Autodesk Inventor part; units mm, degrees
ref_plane "YZ Plane" through (0, 0, 0) normal (1, 0, 0) x (0, 1, 0)
ref_plane "XZ Plane" through (0, 0, 0) normal (0, 1, 0) x (-1, 0, 0)
ref_plane "XY Plane" through (0, 0, 0) normal (0, 0, 1) x (1, 0, 0)
sketch "Sketch1" plane through (0, 0, 0) normal (0, 0, 1) x (1, 0, 0)
  line L0 (-12.7, 25.4) -> (12.7, 25.4)
  line L1 (12.7, 25.4) -> (12.7, -25.4)
  line L2 (12.7, -25.4) -> (-12.7, -25.4)
  line L3 (-12.7, -25.4) -> (-12.7, 25.4)
  line L4 (-12.7, 25.4) -> (12.7, -25.4) construction
  line L5 (12.7, 25.4) -> (-12.7, -25.4) construction
  line L6 (-33.3465, 77.1501) -> (5.5685, 44.4965)
  line L7 (5.5685, 44.4965) -> (-10.7583, 25.039)
  line L8 (-10.7583, 25.039) -> (-49.6733, 57.6926)
  line L9 (-49.6733, 57.6926) -> (-33.3465, 77.1501)
  line L10 (-33.3465, 77.1501) -> (-10.7583, 25.039) construction
  line L11 (5.5685, 44.4965) -> (-49.6733, 57.6926) construction
  line L12 (-31.7812, 59.258) -> (-12.3236, 42.9312) construction
  line L13 (0, -12.7) -> (0, 12.7) construction
  line L14 (-12.7, -25.4) -> (12.7, -25.4)
  line L15 (12.7, -25.4) -> (12.7, -50.8)
  line L16 (12.7, -50.8) -> (-12.7, -50.8)
  line L17 (-12.7, -50.8) -> (-12.7, -25.4)
  circle A0 centre (0, -38.1) radius 12.7
  circle A1 centre (-31.7812, 59.258) radius 12.7
  line L18 (-10.7583, 25.039) -> (-185.876, 171.9802)
  arc A2 (-12.7, 25.4) -> (-13.6716, 27.4835) centre (-15.4199, 25.4) ccw
  arc A3 (12.7, 25.4) -> (5.5685, 44.4965) centre (-16.4339, 25.4) ccw
  circle A4 centre (0, -12.7) radius 12.7
  point P0 (0, 0)
  point P1 (0, 0)
  point P2 (0, 0)
  point P3 (-22.0524, 51.0946)
  point P4 (-22.0524, 51.0946)
  point P5 (-39.9446, 49.5292)
  point P6 (-12.7, -38.1)
  point P7 (12.7, -38.1)
  point P8 (-23.6178, 68.9867)
  point P9 (-10.4554, 25.4)
  point P10 (-11.1885, 25.4)
  point P11 (-41.5099, 67.4214)
  point P12 (-39.9446, 49.5292)
  point P13 (-13.6716, 27.4835)
  point P14 (-11.1885, 25.4)
  point P15 (12.7, -12.7)
  point P16 (-12.7, -12.7)
  dimension "d0" = 25.4
  dimension "d1" = 50.8
  dimension "d2" = 25.4
  dimension "d3" = 12.7
  dimension "d14" = 25.4
extrude "Extrusion1" add sketch "Sketch1" along normal blind 3.175 contours A2 L8 L0 | L0 L8 L7 L1 A4 L3 | L8 A1 L6 L7 L0 | L0 L7 L8 | A4 | L7 A3 L0 | A1
hole "Hole1" at (0, -12.7, 0) at (0, 12.7, 0) at (-12.3236, 42.9312, 0) at (-31.7812, 59.258, 0) at (0, -38.1, 0) direction (0, 0, 1) diameter 4.445 end through all
properties part number "Hood Lower Bracket" material "PET Plastic"
Check sheet for the modelled part. Datum: model origin and axes. Units: mm. A direction names the side the tool comes from. Round coordinates to 2 decimals unless told otherwise and drop trailing zeros. Loops run counter-clockwise (first coordinate to the right, second up) from the corner with the lowest first, then second, coordinate; pieces in that order, holes last. Notation, with made-up numbers: M -4.75,-28.5 L 45.25,-28.5 A17 cw 45.25,-14.5 Z; hole C -11.5,49.5 d10. An arc over 180 degrees is marked long. One line per question, with ' | ' between items. Start each with the question number.
Item 1: Section check C-C (z = 2.2). Record the boundary of the cut face in (x, y) (1 decimal), and give its area (3 significant figures).
Item 2: Section check B-B (x = 0). Record the boundary of the cut face in (y, z) (1 decimal).
Item 3: Set-up check for faces 5 (the face through (-12.7, 6, 2)), 6 (the face through (-41.687, 67.206, 1.565)): record each of +Z, -Z, +X, -X, +Y, -Y from which the full face is reachable in a straight line by a thin tool's end or side.
Item 4: Section check D-D (y = -14). Record the boundary of the cut face in (x, z) (3 decimals), and give its area (3 significant figures).
Item 5: Gauge pin test, flat ends, axial feed: pin 1 Ø3.5 at (x, y) = (0, 12.7) entering from +Z; pin 2 Ø1.6 at (y, z) = (0, 1) entering from -X; pin 3 Ø7 at (x, y) = (-31.78, 59.26) entering from -Z. Record the tip position at first contact, or that the pin passes through.
Item 6: Scan lines: probe 1 along X at (y, z) = (-12.7, 1.95); probe 2 along Y at (x, z) = (0, 2); probe 3 along Y at (x, z) = (-1.5, 1.8). Record each from-to range of solid material in increasing order.
Item 7: Section check A-A (y = 12.7). Record the boundary of the cut face in (x, z) (1 decimal), and give its area (3 significant figures).
Item 8: Release check for a two-part mould opening along Y. For faces 1 (the face through (-12.42, 40.71, 1.61)), 2 (the face through (10.808, 35.729, 1.565)), 3 (the face through (-10, 24, 0)), 4 (the face through (0.279, -25.397, 1.565)) record: released by +Y, released by -Y, zero draft, split by the parting line, or undercut.
Worked out:
1) outline: M -39.9,49.5 L -13.7,27.5 A2.7 cw -12.7,25.4 L -12.7,-12.7 A12.7 ccw 12.7,-12.7 L 12.7,25.4 A29.1 ccw 5.6,44.5 L -23.6,69 A12.7 ccw Z; hole C -31.8,59.3 d4.4; hole C -12.3,42.9 d4.4; hole C 0,-12.7 d4.4; hole C 0,12.7 d4.4 | area: 2,630 mm^2
2) outline: M -25.4,0 L -14.9,0 L -14.9,3.2 L -25.4,3.2 Z; M -10.5,0 L 10.5,0 L 10.5,3.2 L -10.5,3.2 Z; M 14.9,0 L 49.2,0 L 49.2,3.2 L 14.9,3.2 Z
3) face 5: +Z, -Z, -X, -Y | face 6: +Z, -Z
4) outline: M -12.633,0 L -1.803,0 L -1.803,3.175 L -12.633,3.175 Z; M 1.803,0 L 12.633,0 L 12.633,3.175 L 1.803,3.175 Z | area: 68.8 mm^2
5) pin 1: through | pin 2: x = -12.7 | pin 3: z = 0
6) probe 1: -12.7 to -2.22, 2.22 to 12.7 | probe 2: -25.4 to -14.92, -10.48 to 10.48, 14.92 to 49.17 | probe 3: -25.31 to -14.34, -11.06 to 11.06, 14.34 to 50.43
7) outline: M -12.7,0 L -2.2,0 L -2.2,3.2 L -12.7,3.2 Z; M 2.2,0 L 12.7,0 L 12.7,3.2 L 2.2,3.2 Z | area: 66.5 mm^2
8) face 1: undercut | face 2: released by +Y | face 3: zero draft | face 4: released by -Y
